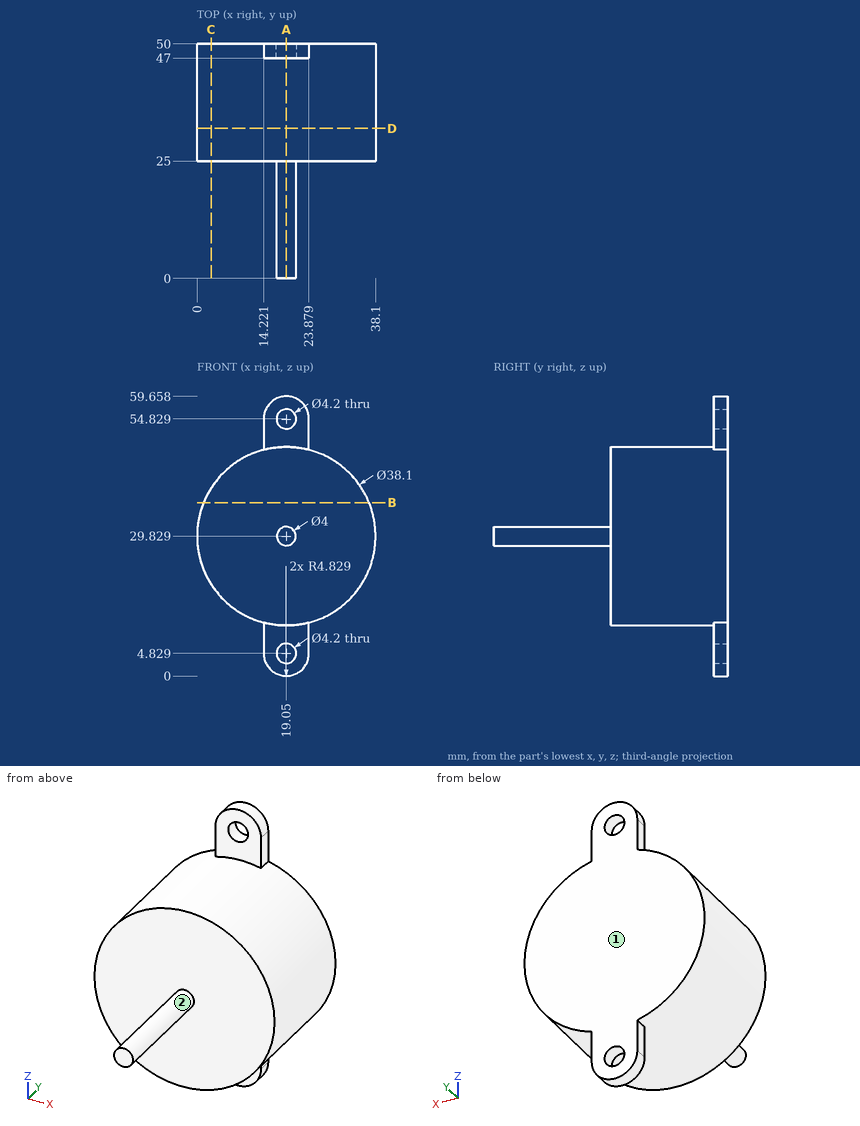
Verification items for this drawing (mm, ordinates from the low corner). A direction names the side the tool comes from. Give positions to 0.01 mm unless a question says otherwise; leave off trailing zeros. Loops run counter-clockwise (first coordinate to the right, second up) from the corner with the lowest first, then second, coordinate; pieces in that order, holes last. Notation, with made-up numbers: M 65,9 L 108,9 A17 ccw 108,34 Z; hole C 27,78.5 d9. An arc over 180 degrees is marked long. Write item = value, one per line. Start each with the question number.
1. Tool access check on the marked faces 1 and 2. Record the directions out of +Z, -Z, +X, -X, +Y, -Y that give a thin tool (end or side, any length) a straight path to the whole face; none if there is none.
2. Thickness scan on probe 1 along Z at (x, y) = (19.05, 48.3); probe 2 along Y at (x, z) = (19.5, 8.5); probe 3 along Y at (x, z) = (28.5, 27.5). Record the ranges inside material, lowest first.
3. Section check B-B, the plane z = 37. Enter the section's corners in (x, y).
4. Section check C-C, the plane x = 3. Enter the section's corners in (y, z), plus the area to 3 significant figures.
5. Section check A-A, the plane x = 19.05. Enter the section's corners in (y, z).
6. Go/stop test with flat-tipped pins: P1, Ø3, axis at x = 21, z = 53, coming from the -Y side; P2, Ø2.5, axis at y = 48.5, z = 7.5, coming from the +X side; P3, Ø6, axis at y = 9.5, z = 26, coming from the -X side. Record where each tip stops, or that it passes through.
7. Section check D-D, the plane y = 32. Enter the section's corners in (x, z).
Values follow:
q1.face_1 = +Z, -Z, +X, -X, +Y
q1.face_2 = -Y
q2.probe_1 = 0 to 2.73, 6.93 to 52.73, 56.93 to 59.66
q2.probe_2 = 47 to 50
q2.probe_3 = 25 to 50
q3.outline = M 1.4,25 L 36.7,25 L 36.7,50 L 1.4,50 Z
q4.outline = M 25,19.57 L 50,19.57 L 50,40.09 L 25,40.09 Z
q4.area = 513 mm^2
q5.outline = M 0,27.83 L 25,27.83 L 25,10.78 L 47,10.78 L 47,6.93 L 50,6.93 L 50,52.73 L 47,52.73 L 47,48.88 L 25,48.88 L 25,31.83 L 0,31.83 Z; M 47,0 L 50,0 L 50,2.73 L 47,2.73 Z; M 47,56.93 L 50,56.93 L 50,59.66 L 47,59.66 Z
q6.P1 = 47
q6.P2 = 23.88
q6.P3 = 17.23
q7.outline = C 19.05,29.83 d38.1
